The listing builds one solid part. Answer for the finished solid, in the listing's coordinates (mm). A direction names the side the tool comes from. Coordinates: 2 decimals unless noted, no trailing zeros. Loops run counter-clockwise (first coordinate to the right, second up) from the corner with the lowest first, then second, coordinate; pieces in that order, holes last. Notation, with made-up numbers: M 34.25,19.25 L 76.25,19.25 A18 cw 76.25,42.25 Z; hole C 18.25,20.25 d1. An arc over 180 degrees is marked long. Return JSON: item names as keys, results as strings. Group by question number.
1. Section C-C (x = -32) is taken. Write down the section's boundary in (y, z), then the cut area to 3 significant figures.
2. Given P1, Ø2, axis at y = 11, z = -5.5, coming from the +X side; P2, Ø19.5, axis at x = -1.5, z = -46.5, coming from the +Y side; P3, Ø2, axis at y = 8, z = -65.5, coming from the -X side, each flat-ended and moving along its own axis, determine where each tip first touches the part or whether it passes through.
3. Which of the six approach directions +Z, -Z, +X, -X, +Y, -Y give full straight-line access (tool end or side, diameter ignored) to faces 1 (the face through (8.89, -24, -34)), 2 (the face through (1.27, 8, -64)), 3 (the face through (-8.89, -24, -47))?
4. Section B-B (z = -48.26) is taken. Write down the section's boundary in (x, y), then the cut area to 3 significant figures.
5. The mould has two halves that part along Y. Classify faces 4 (the face through (6.66, 5.89, -64.72)), 5 (the face through (-31.6, -8.5, -1.778)), 6 (the face through (-1.27, 8, -64)): pulls with the +Y half, pulls with the -Y half, needs draft (parallel to the pull), parting line crosses it, or undercut.
6. Section D-D (y = 2) is taken. Count the separate pieces of the cut face and the enclosed holes in it, then the cut area to 3 significant figures.
7. Straight lines are drawn through the part: L1, parallel to Z at x = 0, y = -26; L2, parallel to Z at x = 4, y = -22; L3, parallel to X at y = -25.3, z = -48.26. For each, find the intervals that lie inside material, in ascending order. Write a range as from..to.
8. Section A-A (x = 0) is taken. Write down the section's boundary in (y, z), then the cut area to 3 significant figures.
```python
from build123d import *

# Parameters (mm, degrees)
SKETCH1_W                = 4.064
SKETCH1_H                = 13.843
BOSS_EXTRUDE1_DEPTH      = 7.62
BOSS_EXTRUDE2_START      = -1.778
BOSS_EXTRUDE2_DEPTH      = 1.778
BOSS_EXTRUDE3_DEPTH      = 1.778
SKETCH4_W                = 17.78
SKETCH4_H                = 4.445
BOSS_EXTRUDE4_DEPTH      = 60.96
BOSS_EXTRUDE5_START      = -7.62
BOSS_EXTRUDE5_DEPTH      = 7.62
M3_CLEARANCE_HOLE1_D     = 3.6
M3_CLEARANCE_HOLE1_DEPTH = 25.4
M3_CLEARANCE_HOLE1_TIP   = 1.081549114


with BuildPart() as part:
    # Sketch1 → Boss-Extrude1 (new body)
    with BuildSketch(Plane.XY):
        with BuildLine():
            Line((-38.354, -27.686), (-12.954, -27.686))
            Line((-12.954, -27.686), (-12.954, -13.843))
            Line((-12.954, -13.843), (-12.954, 0))
            ThreePointArc((-12.954, 0), (-25.654, -12.7), (-38.354, 0))
            Line((-38.354, 0), (-38.354, -27.686))
        make_face()
        with BuildLine():
            Line((8.89, -27.686), (8.89, 0))
            ThreePointArc((8.89, 0), (0, -8.89), (-8.89, 0))
            Line((-8.89, 0), (-8.89, -13.843))
            Line((-8.89, -13.843), (-8.89, -27.686))
            Line((-8.89, -27.686), (8.89, -27.686))
        make_face()
        with BuildLine():
            ThreePointArc((-8.89, 0), (0, -8.89), (8.89, 0))
            Line((8.89, 0), (7.62, 0))
            ThreePointArc((7.62, 0), (0, -7.62), (-7.62, 0))
            Line((-7.62, 0), (-8.89, 0))
        make_face()
        with BuildLine():
            ThreePointArc((-1.27, 8.798818102), (-6.72020833, 5.819871133), (-8.89, 0))
            Line((-8.89, 0), (-7.62, 0))
            ThreePointArc((-7.62, 0), (-5.819871133, 4.91868885), (-1.27, 7.513421325))
            Line((-1.27, 7.513421325), (-1.27, 8.798818102))
        make_face()
        with BuildLine():
            Line((7.62, 0), (8.89, 0))
            ThreePointArc((8.89, 0), (6.72020833, 5.819871133), (1.27, 8.798818102))
            Line((1.27, 8.798818102), (1.27, 7.513421325))
            ThreePointArc((1.27, 7.513421325), (5.819871133, 4.91868885), (7.62, 0))
        make_face()
        with BuildLine():
            ThreePointArc((-38.354, 0), (-25.654, -12.7), (-12.954, 0))
            Line((-12.954, 0), (-14.224, 0))
            ThreePointArc((-14.224, 0), (-25.654, -11.43), (-37.084, 0))
            Line((-37.084, 0), (-38.354, 0))
        make_face()
        with BuildLine():
            Line((-14.224, 0), (-12.954, 0))
            ThreePointArc((-12.954, 0), (-15.816622301, 8.032185257), (-23.114, 12.443407893))
            Line((-23.114, 12.443407893), (-23.114, 11.144204772))
            ThreePointArc((-23.114, 11.144204772), (-16.718757978, 7.127857322), (-14.224, 0))
        make_face()
        with BuildLine():
            ThreePointArc((-28.194, 12.443407893), (-35.491377699, 8.032185257), (-38.354, 0))
            Line((-38.354, 0), (-37.084, 0))
            ThreePointArc((-37.084, 0), (-34.589242022, 7.127857322), (-28.194, 11.144204772))
            Line((-28.194, 11.144204772), (-28.194, 12.443407893))
        make_face()
        with Locations((-10.922, -20.7645)):
            Rectangle(SKETCH1_W, SKETCH1_H)
    extrude(amount=-BOSS_EXTRUDE1_DEPTH)

    # Sketch2 → Boss-Extrude2 (add)
    with BuildSketch(Plane(origin=(0, 0, -7.62), x_dir=(-1, 0, 0), z_dir=(0, 0, -1)).offset(BOSS_EXTRUDE2_START)):
        with BuildLine():
            Line((-1.27, 6.221703947), (-1.27, 7.513421325))
            ThreePointArc((-1.27, 7.513421325), (-4.91868885, -5.819871133), (7.62, 0))
            ThreePointArc((7.62, 0), (5.819871133, 4.91868885), (1.27, 7.513421325))
            Line((1.27, 7.513421325), (1.27, 6.221703947))
            ThreePointArc((1.27, 6.221703947), (4.91868885, 4.016092628), (6.35, 0))
            ThreePointArc((6.35, 0), (-4.016092628, -4.91868885), (-1.27, 6.221703947))
        make_face()
    boss_extrude2 = extrude(amount=BOSS_EXTRUDE2_DEPTH)

    # Sketch3 → Boss-Extrude3 (add)
    with BuildSketch(Plane.XY):
        with BuildLine():
            Line((-28.194, 9.837377699), (-28.194, 11.144204772))
            ThreePointArc((-28.194, 11.144204772), (-32.781857322, -8.935242022), (-14.224, 0))
            ThreePointArc((-14.224, 0), (-16.718757978, 7.127857322), (-23.114, 11.144204772))
            Line((-23.114, 11.144204772), (-23.114, 9.837377699))
            ThreePointArc((-23.114, 9.837377699), (-17.621814743, 6.221703947), (-15.494, 0))
            ThreePointArc((-15.494, 0), (-31.875703947, -8.032185257), (-28.194, 9.837377699))
        make_face()
    extrude(amount=-BOSS_EXTRUDE3_DEPTH)

    # Sketch4 → Boss-Extrude4 (add)
    with BuildSketch(Plane(origin=(0, 0, -7.62), x_dir=(-1, 0, 0), z_dir=(0, 0, -1))):
        with Locations((0, -25.4635)):
            Rectangle(SKETCH4_W, SKETCH4_H)
    extrude(amount=BOSS_EXTRUDE4_DEPTH)

    # Sketch5 → Boss-Extrude5 (add)
    with BuildSketch(Plane(origin=(0, 0, -68.58), x_dir=(-1, 0, 0), z_dir=(0, 0, -1)).offset(BOSS_EXTRUDE5_START)):
        with BuildLine():
            Line((8.89, -23.241), (8.89, 0))
            ThreePointArc((8.89, 0), (0, -8.89), (-8.89, 0))
            Line((-8.89, 0), (-8.89, -23.241))
            Line((-8.89, -23.241), (8.89, -23.241))
        make_face()
        with BuildLine():
            ThreePointArc((-8.89, 0), (0, -8.89), (8.89, 0))
            ThreePointArc((8.89, 0), (6.72020833, 5.819871133), (1.27, 8.798818102))
            Line((1.27, 8.798818102), (1.27, 7.513421325))
            ThreePointArc((1.27, 7.513421325), (5.819871133, 4.91868885), (7.62, 0))
            ThreePointArc((7.62, 0), (-4.91868885, -5.819871133), (-1.27, 7.513421325))
            Line((-1.27, 7.513421325), (-1.27, 8.798818102))
            ThreePointArc((-1.27, 8.798818102), (-6.72020833, 5.819871133), (-8.89, 0))
        make_face()
    extrude(amount=BOSS_EXTRUDE5_DEPTH)

    # Mirror1: Boss-Extrude2 across plane
    add(boss_extrude2.mirror(Plane(origin=(0, 0, -34.29), x_dir=(1, 0, 0), z_dir=(0, 0, -1))))

    # M3 Clearance Hole1
    with Locations(Plane(origin=(0, -23.241, 0), x_dir=(1, 0, 0), z_dir=(0, 1, 0))):
        with Locations((0, 20.32), (0, 48.26)):
            Hole(M3_CLEARANCE_HOLE1_D / 2, depth=M3_CLEARANCE_HOLE1_DEPTH)
            with Locations((0, 0, -(M3_CLEARANCE_HOLE1_DEPTH + M3_CLEARANCE_HOLE1_TIP / 2))):  # 118° drill point
                Cone(0, M3_CLEARANCE_HOLE1_D / 2, M3_CLEARANCE_HOLE1_TIP, mode=Mode.SUBTRACT)


solid = part.part
```
Worked out:
{
 "1": {"outline": "M -27.69,-7.62 L -9.51,-7.62 L -9.51,-1.78 L -7.93,-1.78 L -7.93,0 L -27.69,0 Z; M 7.93,-1.78 L 9.51,-1.78 L 9.51,-7.62 L 11,-7.62 L 11,0 L 7.93,0 Z", "area": "156 mm^2"},
 "2": {"P1": "x = -17.83", "P2": "y = -23.24", "P3": "x = -5.48"},
 "3": {"face 1": "+Z, -Z, +X, +Y, -Y", "face 2": "+Z, -Z, +Y", "face 3": "-Z, -X, +Y, -Y"},
 "4": {"outline": "M -8.89,-27.69 L -1.8,-27.69 L -1.8,-23.24 L -8.89,-23.24 Z; M 1.8,-27.69 L 8.89,-27.69 L 8.89,-23.24 L 1.8,-23.24 Z", "area": "63.0 mm^2"},
 "5": {"face 4": "pulls with the +Y half", "face 5": "undercut", "face 6": "needs draft"},
 "6": {"separate pieces": "6", "enclosed holes": "0", "area": "73.6 mm^2"},
 "7": {"L1": "-68.58..-50.06, -46.46..-22.12, -18.52..0", "L2": "-68.58..-60.96, -7.62..0", "L3": "-8.89..-1.8, 1.8..8.89"},
 "8": {"outline": "M -27.69,-68.58 L -7.62,-68.58 L -7.62,-62.74 L -6.35,-62.74 L -6.35,-60.96 L -23.24,-60.96 L -23.24,-50.06 L -27.69,-50.06 Z; M -27.69,-46.46 L -23.24,-46.46 L -23.24,-22.12 L -27.69,-22.12 Z; M -27.69,-18.52 L -23.24,-18.52 L -23.24,-7.62 L -6.35,-7.62 L -6.35,-5.84 L -7.62,-5.84 L -7.62,0 L -27.69,0 Z", "area": "515 mm^2"}
}
